For this review, take the finished solid that the model builds, in its own axes (mm). Coordinates: 2 decimals unless noted, no trailing zeros. Loops run counter-clockwise (first coordinate to the right, second up) from the corner with the lowest first, then second, coordinate; pieces in that order, holes last. Notation, with made-up numbers: M 3,51.25 L 45,51.25 A17 ccw 45,57.25 Z; hole C -30,40 d8. An arc over 180 degrees is marked long. Answer as a JSON object with one key per item and string values. Group by question number.
Item 1: Add section A-A (z = -206.7). State the section outline as (x, y) points.
Item 2: Wall thickness on L1, parallel to X at y = 1.3, z = -50; L2, parallel to X at y = 1.45, z = -30; L3, parallel to Z at x = -23, y = 2.4: over which ranges is each line inside the solid? List them lowest first. Write a range as from..to.
Item 3: Insertion check: pin 1 (5.5 mm diameter, centred on x = -41.5, z = -215, fed in from -Y); pin 2 (4 mm diameter, centred on x = 41.5, z = -195, fed in from +Y). Each pin has a flat end and moves straight along its axis. Give the tip position at first contact, or say it passes through.
Item 4: Mouldability with a two-part tool opening along Z and no side actions: class faces 1 (the face through (18.4, 1.48, -209.56)), 2 (the face through (1, 3, -78)), 3 (the face through (-16.6, 1.48, -209.56)) as +Z half, -Z half, draft (parallel to the pull), parting line (faces both ways), or undercut.
from build123d import *

# Parameters (mm, degrees)
SKETCH1_W           = 100
SKETCH1_H           = 120
SKETCH1_R           = 2.1
SKETCH1_R_2         = 1.75
BOSS_EXTRUDE1_DEPTH = 3
SKETCH2_R           = 2.1
CUT_EXTRUDE1_DEPTH  = 10
SKETCH3_W           = 100
SKETCH3_H           = 3
BOSS_EXTRUDE2_DEPTH = 160
SKETCH4_R           = 3
SKETCH4_R_2         = 2.1
CUT_EXTRUDE2_DEPTH  = 160


with BuildPart() as part:
    # Sketch1 → Boss-Extrude1 (new body)
    with BuildSketch(Plane(origin=(0, 0, 0), x_dir=(1, 0, 0), z_dir=(0, 1, 0))):
        Rectangle(SKETCH1_W, SKETCH1_H)
        with Locations(Location((41.5, 50, 0), (0, 0, 270))):
            Circle(SKETCH1_R, mode=Mode.SUBTRACT)
        with Locations(Location((41.5, -50, 0), (0, 0, 90))):
            Circle(SKETCH1_R, mode=Mode.SUBTRACT)
        with Locations(Location((-41.5, -50, 0), (0, 0, 270))):
            Circle(SKETCH1_R, mode=Mode.SUBTRACT)
        with Locations(Location((-41.5, 50, 0), (0, 0, 90))):
            Circle(SKETCH1_R, mode=Mode.SUBTRACT)
        with Locations(Location((-42, 30, 0), (0, 0, 270))):
            Circle(SKETCH1_R_2, mode=Mode.SUBTRACT)
        with Locations(Location((0, 30, 0), (0, 0, 270))):
            Circle(SKETCH1_R_2, mode=Mode.SUBTRACT)
        with Locations(Location((42, 30, 0), (0, 0, 270))):
            Circle(SKETCH1_R_2, mode=Mode.SUBTRACT)
    extrude(amount=BOSS_EXTRUDE1_DEPTH)

    # Sketch2 → Cut-Extrude1 (cut)
    with BuildSketch(Plane.XZ):
        with Locations(Location((-24.5, -50, 0), (0, 0, 270))):
            Circle(SKETCH2_R)
        with Locations(Location((24.5, -50, 0), (0, 0, 270))):
            Circle(SKETCH2_R)
        with Locations(Location((24.5, 50, 0), (0, 0, 270))):
            Circle(SKETCH2_R)
        with Locations(Location((-24.5, 50, 0), (0, 0, 270))):
            Circle(SKETCH2_R)
    extrude(amount=-CUT_EXTRUDE1_DEPTH, mode=Mode.SUBTRACT)

    # Sketch3 → Boss-Extrude2 (add)
    with BuildSketch(Plane(origin=(0, 0, -60), x_dir=(-1, 0, 0), z_dir=(0, 0, -1))):
        with Locations((0, 1.5)):
            Rectangle(SKETCH3_W, SKETCH3_H)
    extrude(amount=BOSS_EXTRUDE2_DEPTH)

    # Sketch4 → Cut-Extrude2 (cut)
    with BuildSketch(Plane.XZ):
        with Locations(Location((17.5, -206.7, 0), (0, 0, 270))):
            Circle(SKETCH4_R)
        with Locations(Location((-17.5, -206.7, 0), (0, 0, 270))):
            Circle(SKETCH4_R)
        with Locations(Location((-41.5, -215, 0), (0, 0, 270))):
            Circle(SKETCH4_R_2)
        with Locations(Location((-41.5, -195, 0), (0, 0, 270))):
            Circle(SKETCH4_R_2)
        with Locations(Location((41.5, -195, 0), (0, 0, 270))):
            Circle(SKETCH4_R_2)
        with Locations(Location((41.5, -215, 0), (0, 0, 270))):
            Circle(SKETCH4_R_2)
    extrude(amount=-CUT_EXTRUDE2_DEPTH, mode=Mode.SUBTRACT)


solid = part.part
From the geometry:
{
 "1": {"outline": "M -50,0 L -20.5,0 L -20.5,3 L -50,3 Z; M -14.5,0 L 14.5,0 L 14.5,3 L -14.5,3 Z; M 20.5,0 L 50,0 L 50,3 L 20.5,3 Z"},
 "2": {"L1": "x = -50..-43.6, -39.4..-26.6, -22.4..22.4, 26.6..39.4, 43.6..50", "L2": "x = -50..-43.75, -40.25..-1.75, 1.75..40.25, 43.75..50", "L3": "z = -220..-51.47, -48.53..48.53, 51.47..60"},
 "3": {"pin 1": "stops at y = 0", "pin 2": "passes through"},
 "4": {"face 1": "undercut", "face 2": "draft", "face 3": "undercut"}
}
